Could you check a few things on this model? Use its own coordinates, in mm. Face numbers are marked on the shaded views. A direction names the side the tool comes from. Give positions to 0.01 mm unless a question says otherwise; leave off trailing zeros. Loops run counter-clockwise (first coordinate to the right, second up) from the corner with the lowest first, then second, coordinate; pieces in that order, holes last. Notation, with made-up numbers: (56, 73) - (69, 73) arc R10 cw to (69, 87) - close; hole circle Ø7 at (14, -1). An arc over 180 degrees is marked (long way). Write each question's results on one line, items separated by ' | '. Start each with the question number.
1) I'm going to push flat-ended pins straight in: pin 1 (0.6 mm diameter, centred on y = 31.5, z = -3.5, fed in from +X); pin 2 (1 mm diameter, centred on y = 43.5, z = -7.5, fed in from -X); pin 3 (1 mm diameter, centred on x = 5.5, z = -1, fed in from +Y). Where does each tip first touch, or does it pass through?
2) I want a section at B-B, the plane x = -1.5. Write out the boundary of the cut face in (y, z), and give its area (3 significant figures).
3) If we mould it in two halves opening along X, with no side actions, what happens to the marked faces 4, 5 and 6? For each: +X half, -X half, draft (parallel to the pull), parting line (faces both ways), or undercut.
4) I want a section at D-D, the plane z = 1. Count the separate pieces of the cut face and the enclosed holes in it, and give its area (3 significant figures).
5) I want a section at C-C, the plane x = 5. Write out the boundary of the cut face in (y, z), and give its area (3 significant figures).
6) If I drill on probe 1 along X at (y, z) = (24, -0.75); probe 2 along X at (y, z) = (17, -5.5); probe 3 along Z at (x, y) = (-6, 17), over which ranges is the centre line in solid material (lowest first)? Write a range as [from, to].
7) On a 3-axis mill with a long thin cutter (end or side, diameter ignored), from which of +Z, -Z, +X, -X, +Y, -Y can I reach the whole of each face in a straight line? I mean the marked faces 1, 2 and 3. Say none if no direction works.
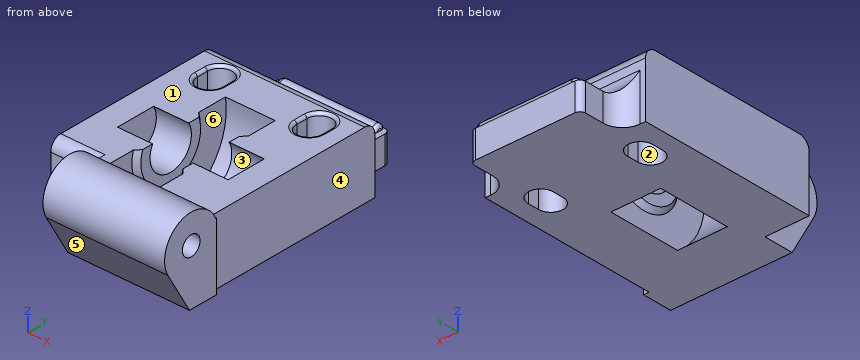
from build123d import *

# Parameters (mm, degrees)
BOSS_EXTRUDE1_DEPTH = 16
SKETCH2_R           = 12
CUT_EXTRUDE1_DEPTH  = 4.5
SKETCH6_R           = 1.75
CUT_EXTRUDE4_DEPTH  = 17.5
BOSS_EXTRUDE2_DEPTH = 0.85
BOSS_EXTRUDE3_START = 0.85
BOSS_EXTRUDE3_DEPTH = 0.85
SKETCH3_R           = 4.12
BEARING_AXIS_DEPTH  = 10
CHAMFER1_SIZE       = 0.85
SKETCH15_W          = 20
SKETCH15_H          = 5
BOSS_EXTRUDE4_DEPTH = 8
FILLET1_R           = 3.5
FILLET3_R           = 1
SKETCH16_R          = 1
BOSS_EXTRUDE5_DEPTH = 9
FILLET4_R           = 0.6
CUT_EXTRUDE8_DEPTH  = 12
FILLET6_R           = 0.5
SKETCH19_W          = 12
SKETCH19_H          = 32.6
CUT_EXTRUDE9_DEPTH  = 1.5
SKETCH20_W          = 12
SKETCH20_H          = 32.6
CUT_EXTRUDE10_DEPTH = 1.5
SKETCH21_W          = 16.964448298
SKETCH21_H          = 10.992811929
CUT_EXTRUDE11_DEPTH = 9.5
SKETCH22_W          = 17.37165941
SKETCH22_H          = 11.278055293
CUT_EXTRUDE12_DEPTH = 0.5
FILLET7_R           = 2


with BuildPart() as part:
    # Sketch1 → Boss-Extrude1 (new, symmetric)
    with BuildSketch(Plane(origin=(0, 0, 0), x_dir=(0, 0, -1), z_dir=(1, 0, 0))):
        with BuildLine():
            Line((10, -0.346), (2.551698211, -4.645302599))
            ThreePointArc((2.551698211, -4.645302599), (-4.784687849, -2.279640803), (-2, 4.908156477))
            Line((-2, 4.908156477), (-2, 37.654))
            Line((-2, 37.654), (10, 37.654))
            Line((10, 37.654), (10, -0.346))
        make_face()
    extrude(amount=BOSS_EXTRUDE1_DEPTH, both=True)

    # Sketch2 → Cut-Extrude1 (cut, symmetric)
    with BuildSketch(Plane(origin=(0, 0, 0), x_dir=(0, 0, -1), z_dir=(1, 0, 0))):
        with Locations((0, 17)):
            Circle(SKETCH2_R)
    extrude(amount=CUT_EXTRUDE1_DEPTH, both=True, mode=Mode.SUBTRACT)

    # Sketch6 → Cut-Extrude4 (cut, symmetric)
    with BuildSketch(Plane(origin=(0, 0, 0), x_dir=(0, 0, -1), z_dir=(1, 0, 0))):
        Circle(SKETCH6_R)
    extrude(amount=CUT_EXTRUDE4_DEPTH, both=True, mode=Mode.SUBTRACT)

    # Sketch8 → Boss-Extrude2 (add)
    with BuildSketch(Plane(origin=(-4.5, 0, 0), x_dir=(0, 0, -1), z_dir=(1, 0, 0))):
        with BuildLine():
            Line((-2, 23.499230724), (-2, 10.500769276))
            ThreePointArc((-2, 10.500769276), (6.8, 17), (-2, 23.499230724))
        make_face()
    extrude(amount=BOSS_EXTRUDE2_DEPTH)

    # Sketch9 → Boss-Extrude3 (add)
    with BuildSketch(Plane.ZY.offset(-4.5).offset(BOSS_EXTRUDE3_START)):
        with BuildLine():
            Line((2, 23.499230724), (2, 10.500769276))
            ThreePointArc((2, 10.500769276), (-6.8, 17), (2, 23.499230724))
        make_face()
    extrude(amount=-BOSS_EXTRUDE3_DEPTH)

    # Sketch3 → bearing_axis (cut, symmetric)
    with BuildSketch(Plane(origin=(0, 0, 0), x_dir=(0, 0, -1), z_dir=(1, 0, 0))):
        with Locations((0, 17)):
            Circle(SKETCH3_R)
    extrude(amount=BEARING_AXIS_DEPTH, both=True, mode=Mode.SUBTRACT)

    # Chamfer1
    chamfer1_edges = [part.edges().sort_by_distance(p)[0] for p in [
        (3.65, 17, -6.8),
        (-3.65, 17, -6.8),
    ]]
    chamfer(chamfer1_edges, length=CHAMFER1_SIZE - 0.0001)  # a hair under: the kernel refuses the full size

    # Sketch15 → Boss-Extrude4 (add)
    with BuildSketch(Plane(origin=(0, 37.654, 0), x_dir=(1, 0, 0), z_dir=(0, 1, 0))):
        with Locations((0, 7.5)):
            Rectangle(SKETCH15_W, SKETCH15_H)
    extrude(amount=BOSS_EXTRUDE4_DEPTH)

    # Fillet1
    fillet1_edges = [part.edges().sort_by_distance(p)[0] for p in [
        (0, 37.654, -5),
        (10, 37.654, -7.5),
        (-10, 37.654, -7.5),
    ]]
    fillet(fillet1_edges, radius=FILLET1_R)

    # Fillet3
    fillet3_edges = [part.edges().sort_by_distance(p)[0] for p in [
        (-10, 45.654, -7.5),
        (10, 45.654, -7.5),
    ]]
    fillet(fillet3_edges, radius=FILLET3_R)

    # Sketch16 → Boss-Extrude5 (add, symmetric)
    with BuildSketch(Plane(origin=(0, 0, 0), x_dir=(0, 0, -1), z_dir=(1, 0, 0))):
        with Locations((5, 44.654)):
            Circle(SKETCH16_R)
    extrude(amount=BOSS_EXTRUDE5_DEPTH, both=True)

    # Fillet4
    fillet4_edges = [part.edges().sort_by_distance(p)[0] for p in [
        (-9, 44.654, -4),
        (9, 44.654, -4),
    ]]
    fillet(fillet4_edges, radius=FILLET4_R)

    # Sketch18 → Cut-Extrude8 (cut)
    with BuildSketch(Plane.XY.offset(-10)):
        with BuildLine():
            Line((-11.25, 30.654), (-11.25, 32.654))
            ThreePointArc((-11.25, 32.654), (-9, 34.904), (-6.75, 32.654))
            Line((-6.75, 32.654), (-6.75, 30.654))
            ThreePointArc((-6.75, 30.654), (-9, 28.404), (-11.25, 30.654))
        make_face()
        with BuildLine():
            Line((11.25, 32.654), (11.25, 30.654))
            ThreePointArc((11.25, 30.654), (9, 28.404), (6.75, 30.654))
            Line((6.75, 30.654), (6.75, 32.654))
            ThreePointArc((6.75, 32.654), (9, 34.904), (11.25, 32.654))
        make_face()
    extrude(amount=CUT_EXTRUDE8_DEPTH, mode=Mode.SUBTRACT)

    # Fillet6
    fillet6_edges = [part.edges().sort_by_distance(p)[0] for p in [
        (-11.25, 31.654, 2),
        (-9, 34.904, 2),
        (-6.75, 31.654, 2),
        (-9, 28.404, 2),
        (11.25, 31.654, 2),
        (9, 28.404, 2),
        (6.75, 31.654, 2),
        (9, 34.904, 2),
    ]]
    fillet(fillet6_edges, radius=FILLET6_R)

    # Sketch19 → Cut-Extrude9 (cut)
    with BuildSketch(Plane(origin=(16, 0, 0), x_dir=(0, 0, -1), z_dir=(1, 0, 0))):
        with Locations((4, 21.354)):
            Rectangle(SKETCH19_W, SKETCH19_H)
    extrude(amount=-CUT_EXTRUDE9_DEPTH, mode=Mode.SUBTRACT)

    # Sketch20 → Cut-Extrude10 (cut)
    with BuildSketch(Plane.ZY.offset(16)):
        with Locations((-4, 21.354)):
            Rectangle(SKETCH20_W, SKETCH20_H)
    extrude(amount=-CUT_EXTRUDE10_DEPTH, mode=Mode.SUBTRACT)

    # Sketch21 → Cut-Extrude11 (cut)
    with BuildSketch(Plane.ZY.offset(16)):
        with Locations((-1.517775851, -0.442405965)):
            Rectangle(SKETCH21_W, SKETCH21_H)
    extrude(amount=-CUT_EXTRUDE11_DEPTH, mode=Mode.SUBTRACT)

    # Sketch22 → Cut-Extrude12 (cut)
    with BuildSketch(Plane(origin=(16, 0, 0), x_dir=(0, 0, -1), z_dir=(1, 0, 0))):
        with Locations((1.314170295, -0.585027646)):
            Rectangle(SKETCH22_W, SKETCH22_H)
    extrude(amount=-CUT_EXTRUDE12_DEPTH, mode=Mode.SUBTRACT)

    # Fillet7
    fillet7_edges = [part.edges().sort_by_distance(p)[0] for p in [
        (0, 37.654, 2),
        (-10.5, 5.054, 2),
    ]]
    fillet(fillet7_edges, radius=FILLET7_R)


solid = part.part
Answers:
1) pin 1: stops at x = 14.5 | pin 2: stops at x = -10 | pin 3: stops at y = 37.65
2) outline: (-4.65, -2.55) - (-0.35, -10) - (10.37, -10) arc R12 cw to (5.17, 2) - (4.91, 2) arc R5.3 ccw (long way) to start; (23.63, -10) - (45.65, -10) - (45.65, -5) arc R1 ccw to (43.65, -5) - (41.15, -5) arc R3.5 cw to (37.65, -1.5) - (37.65, 0) arc R2 ccw to (35.65, 2) - (28.83, 2) arc R12 cw to start; hole circle Ø3.5 at (0, 0) | area: 295 mm2
3) face 4: +X half | face 5: draft | face 6: undercut
4) separate pieces: 2 | enclosed holes: 3 | area: 753 mm2
5) outline: (-4.65, -2.55) - (-0.35, -10) - (45.65, -10) - (45.65, -5) arc R1 ccw to (43.65, -5) - (41.15, -5) arc R3.5 cw to (37.65, -1.5) - (37.65, 0) arc R2 ccw to (35.65, 2) - (20.6, 2) arc R4.12 cw (long way) to (13.4, 2) - (4.91, 2) arc R5.3 ccw (long way) to start; hole circle Ø3.5 at (0, 0) | area: 508 mm2
6) probe 1: x = [-14.5, -4.5], [4.5, 14.5] | probe 2: x = [-14.5, -3.65], [3.65, 14.5] | probe 3: z = [-10, -4.12]
7) face 1: +Z, +X, -X, +Y | face 2: +Z, -Z | face 3: none
